Can you work these out from the model? Positions are in its coordinate system, mm. Give positions to 0.01 mm unless a question says otherwise; leave off trailing zeros. Loops run counter-clockwise (first coordinate to the right, second up) from the corner with the lowest first, then second, coordinate; pieces in that order, holes last. Notation, with made-up numbers: M 46.25,40 L 97.25,40 A20 cw 97.25,49 Z; hole C 53.5,36.25 d8. An arc over 180 degrees is marked long. One line per item, written item: value. Start each with the question number.
from build123d import *

# Parameters (mm, degrees)
ESBO_O2_W                = 136
ESBO_O2_H                = 100
RESSALTO_EXTRUS_O1_DEPTH = 3
ESBO_O3_R                = 2
CORTE_EXTRUS_O2_DEPTH    = 10
ESBO_O5_W                = 50
ESBO_O5_H                = 3
RESSALTO_EXTRUS_O2_DEPTH = 10
ESBO_O6_W                = 50
ESBO_O6_H                = 3
RESSALTO_EXTRUS_O3_DEPTH = 10
ESBO_O7_R                = 2
CORTE_EXTRUS_O3_DEPTH    = 10


with BuildPart() as part:
    # Esboço2 → Ressalto-extrusão1 (new body)
    with BuildSketch(Plane(origin=(0, 0, 0), x_dir=(1, 0, 0), z_dir=(0, 1, 0))):
        with Locations((-68, 50)):
            Rectangle(ESBO_O2_W, ESBO_O2_H)
    extrude(amount=RESSALTO_EXTRUS_O1_DEPTH)

    # Esboço3 → Corte-extrusão2 (cut)
    with BuildSketch(Plane(origin=(0, 3, 0), x_dir=(1, 0, 0), z_dir=(0, 1, 0))):
        with Locations(Location((-128.5, 10, 0), (0, 0, 270))):
            Circle(ESBO_O3_R)
        with Locations(Location((-7.5, 10, 0), (0, 0, 270))):
            Circle(ESBO_O3_R)
        with Locations(Location((-7.5, 90, 0), (0, 0, 270))):
            Circle(ESBO_O3_R)
        with Locations(Location((-128.5, 90, 0), (0, 0, 270))):
            Circle(ESBO_O3_R)
    extrude(amount=-CORTE_EXTRUS_O2_DEPTH, mode=Mode.SUBTRACT)

    # Esboço5 → Ressalto-extrusão2 (add)
    with BuildSketch(Plane(origin=(0, 0, 0), x_dir=(0, 0, -1), z_dir=(1, 0, 0))):
        with Locations((50, 1.5)):
            Rectangle(ESBO_O5_W, ESBO_O5_H)
    extrude(amount=RESSALTO_EXTRUS_O2_DEPTH)

    # Esboço6 → Ressalto-extrusão3 (add)
    with BuildSketch(Plane.ZY.offset(136)):
        with Locations((-50, 1.5)):
            Rectangle(ESBO_O6_W, ESBO_O6_H)
    extrude(amount=RESSALTO_EXTRUS_O3_DEPTH)

    # Esboço7 → Corte-extrusão3 (cut)
    with BuildSketch(Plane(origin=(0, 3, 0), x_dir=(1, 0, 0), z_dir=(0, 1, 0))):
        with Locations(Location((5, 40, 0), (0, 0, 270))):
            Circle(ESBO_O7_R)
        with Locations(Location((5, 60, 0), (0, 0, 270))):
            Circle(ESBO_O7_R)
        with Locations(Location((-141, 60, 0), (0, 0, 270))):
            Circle(ESBO_O7_R)
        with Locations(Location((-141, 40, 0), (0, 0, 270))):
            Circle(ESBO_O7_R)
    extrude(amount=-CORTE_EXTRUS_O3_DEPTH, mode=Mode.SUBTRACT)


solid = part.part
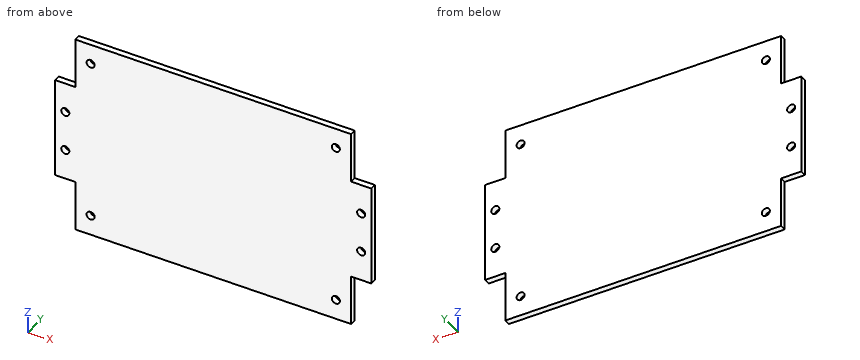
Q1. If we section it at C-C, the plane y = 1.2: Give the number of separate pieces and of enclosed holes in the cut face, plus the area to 3 significant figures.
Q2. I need wall thicknesses on line 1 along X through (y, z) = (2.2, -10); line 2 along Z through (x, y) = (-128.5, 1.15); line 3 along Z through (x, y) = (-141, 1.75). Which ranges of each line are inside material? Lowest first, please.
Q3. If we section it at B-B, the plane x = 5: Write out the boundary of the cut face in (y, z), plus the area to 3 significant figures.
Q4. For P1, Ø1.5, axis at y = 2, z = -80, coming from the -X side; P2, Ø0.9, axis at y = 1.5, z = -88.5, coming from the +X side; P3, Ø0.9, axis at x = -143, y = 1, coming from the +Z side, each with a flat end and sliding along its axis, tell me the tip position at first contact or that it passes through.
Q5. If we section it at D-D, the plane z = -20: Write out the boundary of the cut face in (x, y).
Q6. If we section it at A-A, the plane z = -40: Write out the boundary of the cut face in (x, y), plus the area to 3 significant figures.
Response:
1. separate pieces: 1
1. enclosed holes: 8
1. area: 14,500 mm^2
2. line 1: -136 to -130.5, -126.5 to -9.5, -5.5 to 0
2. line 2: -100 to -92, -88 to -12, -8 to 0
2. line 3: -75 to -62, -58 to -42, -38 to -25
3. outline: M 0,-75 L 3,-75 L 3,-62 L 0,-62 Z; M 0,-58 L 3,-58 L 3,-42 L 0,-42 Z; M 0,-38 L 3,-38 L 3,-25 L 0,-25 Z
3. area: 126 mm^2
4. P1: x = -136
4. P2: x = 0
4. P3: z = -25
5. outline: M -136,0 L 0,0 L 0,3 L -136,3 Z
6. outline: M -146,0 L -143,0 L -143,3 L -146,3 Z; M -139,0 L 3,0 L 3,3 L -139,3 Z; M 7,0 L 10,0 L 10,3 L 7,3 Z
6. area: 444 mm^2
